from build123d import *

# Parameters (mm, degrees)
BOSS_EXTRUDE1_DEPTH     = 20
SKETCH2_R               = 29
CUT_EXTRUDE1_DEPTH      = 1
CUT_EXTRUDE1_DEPTH_BACK = 21
CUT_EXTRUDE2_START      = -16
SKETCH3_R               = 3.25
CUT_EXTRUDE2_DEPTH      = 77


with BuildPart() as part:
    # Sketch1 → Boss-Extrude1 (new body)
    with BuildSketch(Plane.XY):
        with BuildLine():
            Line((-60.5, 0), (60.5, 0))
            Line((60.5, 0), (60.5, 15))
            Line((60.5, 15), (43.5, 15))
            Line((43.5, 15), (32.514998433, 50.938555071))
            ThreePointArc((32.514998433, 50.938555071), (0, 75), (-32.514998433, 50.938555071))
            Line((-32.514998433, 50.938555071), (-43.5, 15))
            Line((-43.5, 15), (-60.5, 15))
            Line((-60.5, 15), (-60.5, 0))
        make_face()
    extrude(amount=BOSS_EXTRUDE1_DEPTH)

    # Sketch2 → Cut-Extrude1 (cut, two sides)
    with BuildSketch(Plane(origin=(0, 0, 0), x_dir=(-1, 0, 0), z_dir=(0, 0, -1))) as cut_extrude1_sk:
        with Locations((0, 41)):
            Circle(SKETCH2_R)
    extrude(amount=CUT_EXTRUDE1_DEPTH, mode=Mode.SUBTRACT)
    extrude(cut_extrude1_sk.sketch, amount=-CUT_EXTRUDE1_DEPTH_BACK, mode=Mode.SUBTRACT)

    # Sketch3 → Cut-Extrude2 (cut)
    with BuildSketch(Plane(origin=(0, 15, 0), x_dir=(1, 0, 0), z_dir=(0, 1, 0)).offset(CUT_EXTRUDE2_START)):
        with Locations((-53, -10)):
            Circle(SKETCH3_R)
    cut_extrude2 = extrude(amount=CUT_EXTRUDE2_DEPTH, mode=Mode.SUBTRACT)

    # Mirror1: Cut-Extrude2 across plane
    add(cut_extrude2.mirror(Plane(origin=(0, 0, 0), x_dir=(0, 0, 1), z_dir=(1, 0, 0))), mode=Mode.SUBTRACT)


solid = part.part
Here's how the part is built. I have some questions about the finished solid (model axes, mm). A direction names the side the tool comes from. Round coordinates to 2 decimals unless told otherwise and drop trailing zeros. Loops run counter-clockwise (first coordinate to the right, second up) from the corner with the lowest first, then second, coordinate; pieces in that order, holes last. Notation, with made-up numbers: (-13, 25.25) - (10, 25.25) arc R9 cw to (10, 33.25) - close; hole circle Ø2 at (65, -28.5). An arc over 180 degrees is marked (long way). One line per question, with ' | ' between items. Start each with the question number.
Q1. I want a section at A-A (x = 53). Write out the boundary of the cut face in (y, z), then the cut area to 4 significant figures.
Q2. Please list where these lines run through material, in increasing order: line 1 (Z direction, x = 53, y = 9.5); line 2 (Y direction, x = 0, z = 7); line 3 (Y direction, x = 3, z = 4.25). Write a range as [from, to].
Q3. Will these pins go through, and if not, where does the flat tip stop? pin 1 (2 mm diameter, centred on x = -46, z = 17, fed in from +Y); pin 2 (8 mm diameter, centred on y = 63, z = 18, fed in from +X); pin 3 (8 mm diameter, centred on y = 31.5, z = 17.5, fed in from -X).
Q4. I want a section at B-B (y = 44.5). Write out the boundary of the cut face in (x, z).
Q5. We'd pull the mould along Z, two halves only. Please class faces 1 (the flat face through (-1, 0, 10)), 2 (the cylindrical face through (-49.9, 7.4, 9.02)), 3 (the flat face through (0, 10, 20)): +Z half, -Z half, draft (parallel to the pull), parting line (faces both ways), or undercut.
Q6. I want a section at C-C (z = 17.75). Write out the boundary of the cut face in (x, y) (3 decimals).
Q7. For faces 4 (the flat face through (0, 10, 0)), 5 (the flat face through (-50, 15, 8)), 6 (the flat face through (50, 15, 8)), which set-ups out of +Z, -Z, +X, -X, +Y, -Y let a thin tool reach every point of the face, with its end or its side?
Q8. I want a section at D-D (x = -38.5). Write out the boundary of the cut face in (y, z).
Response values:
1) outline: (0, 0) - (15, 0) - (15, 6.75) - (0, 6.75) - close; (0, 13.25) - (15, 13.25) - (15, 20) - (0, 20) - close | area: 202.5 mm²
2) line 1: z = [0, 6.75], [13.25, 20] | line 2: y = [0, 12], [70, 75] | line 3: y = [0, 12.16], [69.84, 74.87]
3) pin 1: stops at y = 15 | pin 2: stops at x = 28.84 | pin 3: stops at x = -39.68
4) outline: (-34.48, 0) - (-28.79, 0) - (-28.79, 20) - (-34.48, 20) - close; (28.79, 0) - (34.48, 0) - (34.48, 20) - (28.79, 20) - close
5) face 1: draft | face 2: undercut | face 3: +Z half
6) outline: (-60.5, 0) - (60.5, 0) - (60.5, 15) - (43.5, 15) - (32.515, 50.939) arc R34 ccw to (-32.515, 50.939) - (-43.5, 15) - (-60.5, 15) - close; hole circle Ø58 at (0, 41)
7) face 4: -Z, +X, -X, +Y, -Y | face 5: +Z, -Z, -X, +Y | face 6: +Z, -Z, +X, +Y
8) outline: (0, 0) - (31.36, 0) - (31.36, 20) - (0, 20) - close
